Design review of the part shown in the three views and the two pictorial views. Dimensions are in mm from the part's minimum x, y and z. A direction names the side the tool comes from. Give positions to 0.01 mm unless a question says otherwise; leave off trailing zeros. Write each loop counter-clockwise with the first axis right and the second up, starting at its lowest first coordinate (ties: lowest second). Pieces come first, ordered by that corner, then holes. Notation, with made-up numbers: M 39.5,-36 L 69.5,-36 A20 cw 69.5,-30 Z; hole C 18.5,58 d4. An arc over 180 degrees is marked long. Use one line per item in the form item = value. Start each with the question number.
Q1. Clearance check with flat-ended pins moving along their axes: pin 1 Ø2.5 at (y, z) = (1.5, 59) entering from +X; pin 2 Ø1 at (y, z) = (7.5, 19.5) entering from +X; pin 3 Ø9 at (x, y) = (29, 12) entering from +Z. State where each tip first meets the part, or that it passes through.
Q2. Consider section B-B on y = 1.5. Write out the cut boundary in (x, z), and give its area (3 significant figures).
Q3. Mouldability with a two-part tool opening along X and no side actions: class the marked faces 1 and 2 as released by +X, released by -X, zero draft, split by the parting line, or undercut.
Q4. For probe 1 along Y at (x, z) = (27.5, 22.5); probe 2 along X at (y, z) = (2.5, 56.5); probe 3 along Y at (x, z) = (2.5, 51.5), list the stretches that pass through material, from the lowest coordinate up. Write a range as [from, to].
Q5. Tool access review of the marked faces 3, 4 and 5: name each direction out of +Z, -Z, +X, -X, +Y, -Y from which nothing blocks a thin tool from reaching the whole face with its end or side.
Q6. Consider section D-D on y = 11.5. Write out the cut boundary in (x, z) (1 decimal), and give its area (3 significant figures).
Q7. Consider section A-A on z = 56.5. Write out the cut boundary in (x, y).
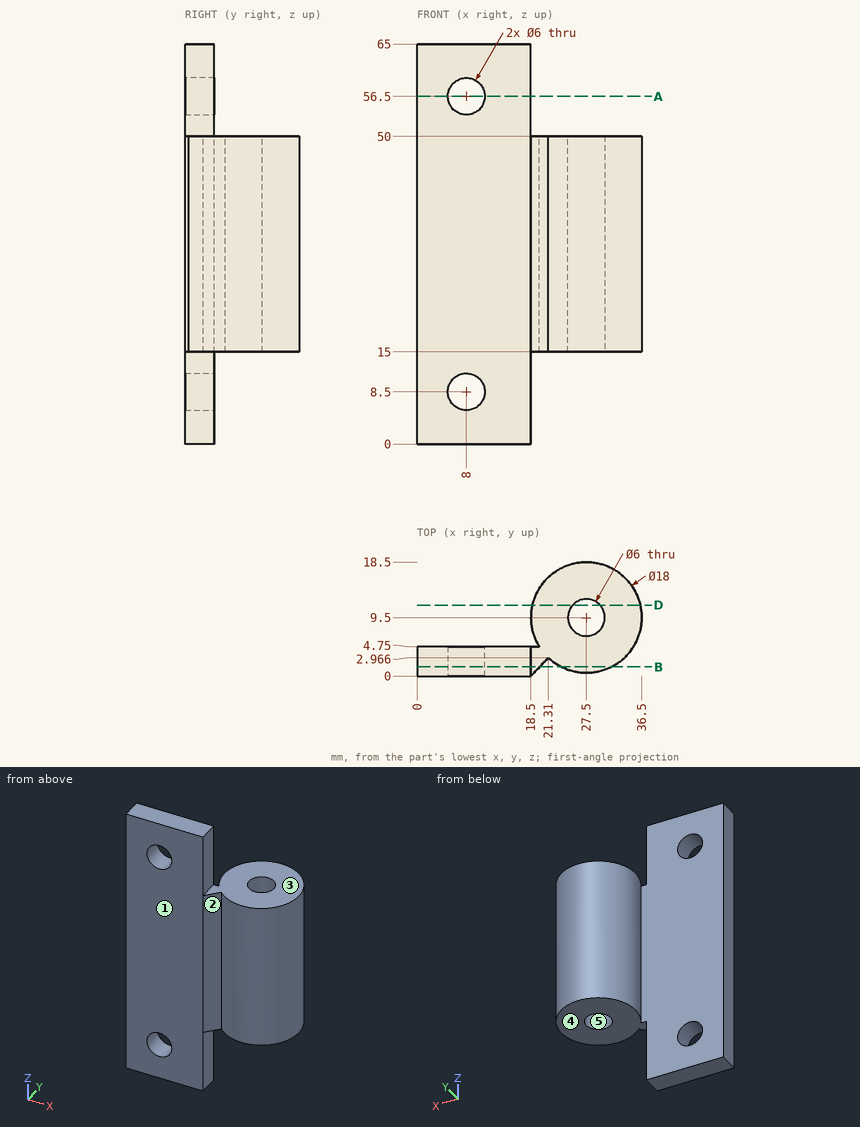
Working result:
q1.pin_1 = 18.5
q1.pin_2 = 36.37
q1.pin_3 = 50
q2.outline = M 0,0 L 18.5,0 L 18.5,15 L 19.92,15 L 19.92,50 L 18.5,50 L 18.5,65 L 0,65 Z; M 23.38,15 L 31.62,15 L 31.62,50 L 23.38,50 Z; hole C 8,8.5 d6; hole C 8,56.5 d6
q2.area = 1,480 mm²
q3.face_1 = zero draft
q3.face_2 = undercut
q4.probe_1 = [0.5, 6.5], [12.5, 18.5]
q4.probe_2 = [0, 5], [11, 18.5]
q4.probe_3 = [0, 4.75]
q5.face_3 = +Z, +X, +Y, -Y
q5.face_4 = -Z, +X, +Y, -Y
q5.face_5 = +Z, -Z
q6.outline = M 18.7,15 L 25.3,15 L 25.3,50 L 18.7,50 Z; M 29.7,15 L 36.3,15 L 36.3,50 L 29.7,50 Z
q6.area = 458 mm²
q7.outline = M 0,0 L 5,0 L 5,4.75 L 0,4.75 Z; M 11,0 L 18.5,0 L 18.5,4.75 L 11,4.75 Z
